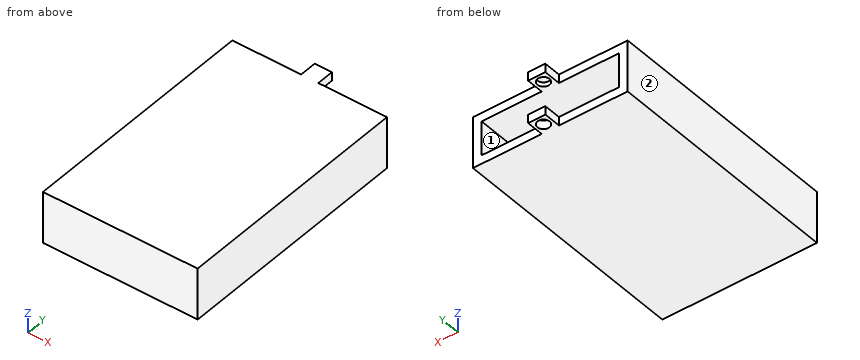
from build123d import *

# Parameters (mm, degrees)
SKETCH1_W           = 90
SKETCH1_H           = 30
BOSS_EXTRUDE1_DEPTH = 140
SKETCH2_W           = 80
SKETCH2_H           = 20
CUT_EXTRUDE1_DEPTH  = 135
SKETCH4_W           = 10
SKETCH4_H           = 30
BOSS_EXTRUDE2_DEPTH = 10
SKETCH7_W           = 20
SKETCH7_H           = 10
CUT_EXTRUDE3_DEPTH  = 10
SKETCH5_R           = 3.5
CUT_EXTRUDE4_DEPTH  = 27.5


with BuildPart() as part:
    # Sketch1 → Boss-Extrude1 (new body)
    with BuildSketch(Plane(origin=(0, 0, 0), x_dir=(1, 0, 0), z_dir=(0, 1, 0))):
        with Locations((-2.788023643, -11.157655047)):
            Rectangle(SKETCH1_W, SKETCH1_H)
    extrude(amount=BOSS_EXTRUDE1_DEPTH)

    # Sketch2 → Cut-Extrude1 (cut)
    with BuildSketch(Plane(origin=(0, 140, 0), x_dir=(1, 0, 0), z_dir=(0, 1, 0))):
        with Locations((-2.788023643, -11.157655047)):
            Rectangle(SKETCH2_W, SKETCH2_H)
    extrude(amount=-CUT_EXTRUDE1_DEPTH, mode=Mode.SUBTRACT)

    # Sketch4 → Boss-Extrude2 (add)
    with BuildSketch(Plane(origin=(0, 140, 0), x_dir=(1, 0, 0), z_dir=(0, 1, 0))):
        with Locations((-2.788023643, -11.157655047)):
            Rectangle(SKETCH4_W, SKETCH4_H)
    extrude(amount=BOSS_EXTRUDE2_DEPTH)

    # Sketch7 → Cut-Extrude3 (cut)
    with BuildSketch(Plane(origin=(2.211976357, 0, 0), x_dir=(0, 0, -1), z_dir=(1, 0, 0))):
        with Locations((-11.157655047, 145)):
            Rectangle(SKETCH7_W, SKETCH7_H)
    extrude(amount=-CUT_EXTRUDE3_DEPTH, mode=Mode.SUBTRACT)

    # Sketch5 → Cut-Extrude4 (cut)
    with BuildSketch(Plane(origin=(0, 0, -3.842344953), x_dir=(-1, 0, 0), z_dir=(0, 0, -1))):
        with Locations((2.788023643, 145)):
            Circle(SKETCH5_R)
    extrude(amount=-CUT_EXTRUDE4_DEPTH, mode=Mode.SUBTRACT)


solid = part.part
Read the model definition and answer for the solid it produces. Units are mm, in the model's axes. Face numbers are marked on the shaded views. A direction names the side the tool comes from. Round coordinates to 2 decimals unless told otherwise and drop trailing zeros. Order: outer loops, then holes, each group sorted by start corner. A loop starts at its lowest first (then second) coordinate and runs counter-clockwise, first axis right, second up.
1) The part is cut by section C-C on z = 7.5. Write down the section's boundary in (x, y), plus the area to 3 significant figures.
2) The part is cut by section A-A on y = 145. Write down the section's boundary in (x, z).
3) Straight lines are drawn through the part: L1, parallel to X at y = 128.5, z = 10; L2, parallel to Z at x = 22.5, y = 129; L3, parallel to X at y = 145, z = 22.4. For each, find the intervals that lie inside material, in ascending order.
4) The part is cut by section D-D on x = 30. Write down the section's boundary in (y, z).
5) Flat-ended cylindrical pins translate along their axes: pin 1 (5.5 mm diameter, centred on y = 147.5, z = 23, fed in from +X); pin 2 (5.5 mm diameter, centred on x = -2.5, y = 145, fed in from -Z); pin 3 (4 mm diameter, centred on y = 145.5, z = -1, fed in from -X). Find the tip coordinate at first contact, or state that the pin passes through.
6) The part is cut by section B-B on y = 46.5. Write down the section's boundary in (x, z).
7) For the marked faces 1 and 2, determine the directions among +Z, -Z, +X, -X, +Y, -Y from which every point of the face is accessible in a straight line to the end or side of a thin tool.
Resolved:
1. outline: (-47.79, 0) - (42.21, 0) - (42.21, 140) - (37.21, 140) - (37.21, 5) - (-42.79, 5) - (-42.79, 140) - (-47.79, 140) - close
1. area: 1,800 mm2
2. outline: (-7.79, -3.84) - (-6.29, -3.84) - (-6.29, 1.16) - (-7.79, 1.16) - close; (-7.79, 21.16) - (-6.29, 21.16) - (-6.29, 23.66) - (0.71, 23.66) - (0.71, 21.16) - (2.21, 21.16) - (2.21, 26.16) - (-7.79, 26.16) - close; (0.71, -3.84) - (2.21, -3.84) - (2.21, 1.16) - (0.71, 1.16) - close
3. L1: x = -47.79 to -42.79, 37.21 to 42.21
3. L2: z = -3.84 to 1.16, 21.16 to 26.16
3. L3: x = -7.79 to -6.29, 0.71 to 2.21
4. outline: (0, -3.84) - (140, -3.84) - (140, 1.16) - (5, 1.16) - (5, 21.16) - (140, 21.16) - (140, 26.16) - (0, 26.16) - close
5. pin 1: stops at x = 2.21
5. pin 2: stops at z = 23.66
5. pin 3: stops at x = -7.79
6. outline: (-47.79, -3.84) - (42.21, -3.84) - (42.21, 26.16) - (-47.79, 26.16) - close; hole (-42.79, 1.16) - (37.21, 1.16) - (37.21, 21.16) - (-42.79, 21.16) - close
7. face 1: +Y
7. face 2: +Z, -Z, -X, +Y, -Y
